Autodesk Inventor part; units mm, degrees
ref_plane "YZ Plane" through (0, 0, 0) normal (1, 0, 0) x (0, 1, 0)
ref_plane "XZ Plane" through (0, 0, 0) normal (0, 1, 0) x (-1, 0, 0)
ref_plane "XY Plane" through (0, 0, 0) normal (0, 0, 1) x (1, 0, 0)
sketch "Boceto1" plane through (0, 0, 0) normal (0, 0, 1) x (1, 0, 0)
  circle A0 centre (0, 0) radius 1.25
  arc A1 (-1.6574, 2.7373) -> (-0.4126, -3.1733) centre (0, 0) ccw
  line L0 (7.1, -4.15) -> (7.1, -7.1226) construction
  line L1 (-3.2, 3.2) -> (-3.2, -3.4) construction
  line L2 (-0.4126, -3.1733) -> (7.1, -4.15)
  line L3 (-1.4, 3.8) -> (-1.4, 6.2978) construction
  line L4 (14.1, 2.7373) -> (14.1, -1.982) construction
  line L5 (7.1, -4.15) -> (8.5447, -4.3189)
  line L6 (8.5447, -4.3189) -> (11.6298, -3.6616)
  line L7 (11.6298, -3.6616) -> (13.3209, -2.1424)
  line L8 (13.9587, -0.9739) -> (13.978, -0.8543)
  line L9 (9.9548, 3.6595) -> (11.6833, 2.9749)
  line L10 (12.6312, 2.1939) -> (13.688, 0.5435)
  arc A2 (12.6312, 2.1939) -> (11.6833, 2.9749) centre (10.9469, 1.1154) ccw
  arc A3 (9.9548, 3.6595) -> (9.2184, 3.8) centre (9.2184, 1.8) ccw
  arc A4 (13.978, -0.8543) -> (13.688, 0.5435) centre (12.0037, -0.535) ccw
  arc A5 (13.3209, -2.1424) -> (13.9587, -0.9739) centre (11.9843, -0.6546) ccw
  line L11 (-1.6574, 2.7373) -> (-2.4537, 3.981)
  line L12 (-2.4537, 3.981) -> (-3.3251, 4.3261)
  line L13 (-3.3251, 4.3261) -> (-3.2, 5.1465)
  line L14 (-3.2, 5.1465) -> (9.2184, 3.8)
  point P0 (9.6, 3.8)
  point P1 (14.1, -0.1)
  dimension "d0" = 2.5
  dimension "d4" = 6.4
  dimension "d5" = 4.15
  dimension "d6" = 10.3
  dimension "d7" = 3.8
  dimension "d8" = 1.8
  dimension "d9" = 11
  dimension "d10" = 7
  dimension "d19" = 2
extrude "Extrusión1" add sketch "Boceto1" along normal blind 1.2
sketch "Boceto5" plane through (0, 0, 1.2) normal (0, 0, 1) x (1, 0, 0)
  line L0 (7.5987, -4.0877) -> (8.5447, -4.3189)
  line L1 (8.5447, -4.3189) -> (11.6298, -3.6616)
  line L2 (11.4934, -3.6907) -> (13.3446, -2.0049)
  line L3 (9.9548, 3.6595) -> (11.6833, 2.9749)
  line L4 (12.6312, 2.1939) -> (13.6823, 0.5523)
  arc A0 (12.6312, 2.1939) -> (11.6833, 2.9749) centre (10.9469, 1.1154) ccw
  arc A1 (9.9548, 3.6595) -> (9.2184, 3.8) centre (9.2184, 1.8) ccw
  arc A2 (13.3446, -2.0049) -> (13.6823, 0.5523) centre (11.998, -0.5262) ccw
  arc A3 (3.8787, -10.625) -> (3.8888, -10.616) centre (2.5421, -9.1373) ccw
  arc A4 (7.5987, -4.0877) -> (7.1292, -0.2455) centre (2.0351, -2.8178) ccw
  arc A5 (7.1292, -0.2455) -> (7.0735, 2.4165) centre (3.9271, 1.0191) ccw
  arc A6 (9.9548, 3.6595) -> (9.2184, 3.8) centre (9.2184, 1.8) ccw
  line L5 (9.2184, 3.8) -> (5.136, 4.2426)
  line L6 (5.136, 4.2426) -> (-1.2086, 4.9306)
  line L7 (9.2184, 3.8) -> (-3.2, 5.1465)
  line L8 (-1.0169, 4.2426) -> (-1.2086, 4.9306)
  line L9 (-1.0169, 4.2426) -> (7.0735, 2.4165)
  point P0 (0, 0)
  point P1 (9.6, 3.8)
extrude "Extrusión5" add sketch "Boceto5" along normal blind 2
sketch "Boceto6" plane through (0, 0, 1.2) normal (0, 0, 1) x (1, 0, 0)
  circle A0 centre (3.427, -1.4569) radius 1.25
  point P0 (0, 0)
  dimension "d26" = 2.5
extrude "Extrusión6" add sketch "Boceto6" along normal blind 3
properties part number "Pieza3_3DPrint"
Build history of the part. All positions in model axes, mm. A direction names the side the tool comes from. Give positions to 0.01 mm unless a question says otherwise; leave off trailing zeros. Order: outer loops, then holes, each group sorted by start corner. A loop starts at its lowest first (then second) coordinate and runs counter-clockwise, first axis right, second up. Notation, with made-up numbers: M 42.5,72.25 L 74.5,72.25 A7 ccw 74.5,78.25 Z; hole C -3,-33.75 d10. An arc over 180 degrees is marked long. Use one line per item in the form item = value.
1) Probe probe 1 along Z at (x, y) = (1.75, -1.75); probe 2 along Y at (x, z) = (0, 0.5); probe 3 along Y at (x, z) = (4.25, 2.1). List the from-to ranges inside material, lowest first.
Calculated:
probe_1 = 0 to 1.2
probe_2 = -3.23 to -1.25, 1.25 to 4.8
probe_3 = -2.4 to -0.52, 3.05 to 4.34
2) Two-plate mould, pull along Y, no slides. Class faces 6 (the face through (12.406, -2.86, 2.186)), 7 (the face through (13.983, -0.769, 2.186)), 8 (the face through (4.62, -1.83, 2.68)): released by +Y, released by -Y, zero draft, split by the parting line, or undercut.
Calculated:
face_6 = released by -Y
face_7 = split by the parting line
face_8 = undercut
3) Tool access for faces 1 (the face through (2.972, 3.342, 2.186)), 2 (the face through (3, 0, 1.2)), 3 (the face through (10.066, -3.995, 1.578)), 4 (the face through (8.065, -4.202, 2.186)), 5 (the face through (-2.88, 4.15, 0.59)): list every direction of +Z, -Z, +X, -X, +Y, -Y with a clear straight run to the whole face (end or side of a thin tool).
Calculated:
face_1 = +Z, -X
face_2 = +Z
face_3 = +Z, -Z, +X, -Y
face_4 = +Z, -X, -Y
face_5 = +Z, -Z, -X
4) Saw through at C-C (x = 0). Give the cut face in (y, z).
Calculated:
outline = M -3.23,0 L -1.25,0 L -1.25,1.2 L -3.23,1.2 Z; M 1.25,0 L 4.8,0 L 4.8,3.2 L 4.01,3.2 L 4.01,1.2 L 1.25,1.2 Z
5) Drop flat-ended pins along their axis: pin 1 (3 mm diameter, centred on x = 12.5, y = -0.5, fed in from +Z); pin 2 (2 mm diameter, centred on y = -1, z = 2.5, fed in from -X); pin 3 (2 mm diameter, centred on y = -2.5, z = 0.5, fed in from -X); pin 4 (2 mm diameter, centred on x = 0, y = 0, fed in from +Z). Give the stop position or say it passes through.
Calculated:
pin_1 = 3.2
pin_2 = 2.18
pin_3 = -2.83
pin_4 = through
6) Saw through at D-D (x = 6.75). Give the cut face in (y, z).
Calculated:
outline = M -4.1,0 L 4.07,0 L 4.07,3.2 L 2.49,3.2 L 2.49,1.2 L -4.1,1.2 Z
